Design review of the part shown in the three views and the two pictorial views. Dimensions are in mm from the part's minimum x, y and z. Round coordinates to 2 decimals unless told otherwise and drop trailing zeros. Loops run counter-clockwise (first coordinate to the right, second up) from the corner with the lowest first, then second, coordinate; pieces in that order, holes last. Notation, with made-up numbers: M 64.5,87.5 L 114.5,87.5 A32 ccw 114.5,121.5 Z; hole C 82,11.25 d1. An arc over 180 degrees is marked long. Answer as CSV lines item,"result". Start each with the question number.
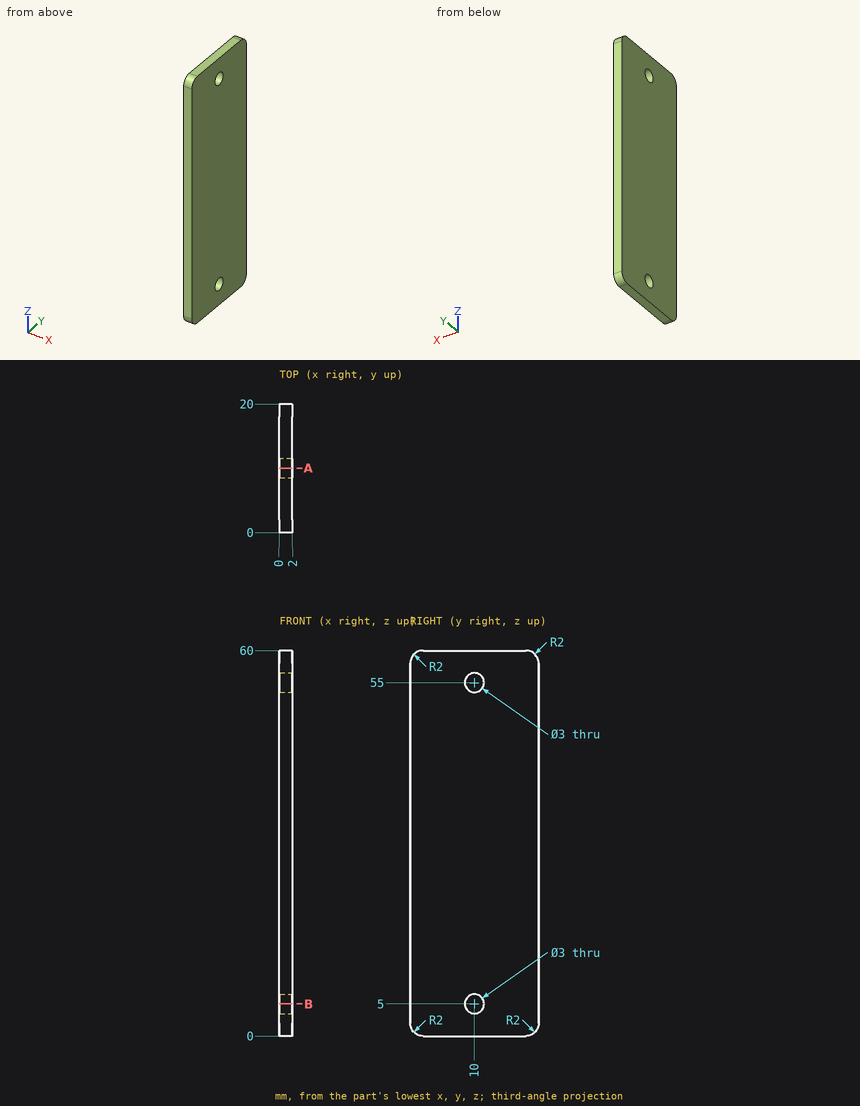
Item 1: Consider section A-A, the plane y = 10. Write out the cut boundary in (x, z), then the cut area to 3 significant figures.
Item 2: Consider section B-B, the plane z = 5. Write out the cut boundary in (x, y).
Item 3: To check wall thickness, follow line 1 (Z direction, x = 1.5, y = 10); line 2 (Y direction, x = 1.65, z = 5.5); line 3 (Y direction, x = 0.5, z = 4). State the ranges of each line that lie inside material, in increasing order.
Item 4: Insertion check: pin 1 Ø2.5 at (y, z) = (10, 55) entering from -X. The pin has a flat end and moves straight along its axis. Give the tip position at first contact, or say it passes through.
Found:
1,outline,"M 0,0 L 2,0 L 2,3.5 L 0,3.5 Z; M 0,6.5 L 2,6.5 L 2,53.5 L 0,53.5 Z; M 0,56.5 L 2,56.5 L 2,60 L 0,60 Z"
1,area,"108 mm^2"
2,outline,"M 0,0 L 2,0 L 2,8.5 L 0,8.5 Z; M 0,11.5 L 2,11.5 L 2,20 L 0,20 Z"
3,line 1,"z = 0 to 3.5, 6.5 to 53.5, 56.5 to 60"
3,line 2,"y = 0 to 8.59, 11.41 to 20"
3,line 3,"y = 0 to 8.88, 11.12 to 20"
4,pin 1,"passes through"
